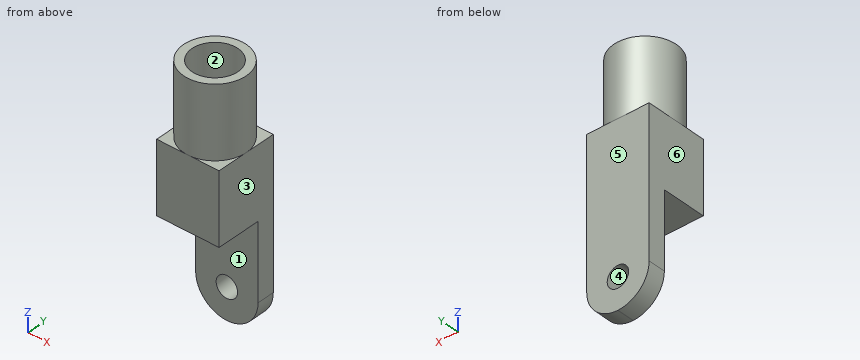
from build123d import *

# Parameters (mm, degrees)
SKETCH1_R           = 4.445
SKETCH1_R_2         = 3.275000003
BOSS_EXTRUDE1_DEPTH = 10.16
SKETCH2_W           = 8.89
SKETCH2_H           = 8.89
BOSS_EXTRUDE2_DEPTH = 25.4
CUT_EXTRUDE1_DEPTH  = 28.275449126
SKETCH4_W           = 15.24
SKETCH4_H           = 6.39064
CUT_EXTRUDE2_DEPTH  = 28.275449126


with BuildPart() as part:
    # Sketch1 → Boss-Extrude1 (new body)
    with BuildSketch(Plane.XY):
        Circle(SKETCH1_R)
        Circle(SKETCH1_R_2, mode=Mode.SUBTRACT)
    extrude(amount=BOSS_EXTRUDE1_DEPTH)

    # Sketch2 → Boss-Extrude2 (add)
    with BuildSketch(Plane(origin=(0, 0, 0), x_dir=(-1, 0, 0), z_dir=(0, 0, -1))):
        Rectangle(SKETCH2_W, SKETCH2_H)
    extrude(amount=BOSS_EXTRUDE2_DEPTH)

    # Sketch3 → Cut-Extrude1 (cut, through all)
    with BuildSketch(Plane.XZ.offset(4.445)):
        with BuildLine():
            Line((4.445, -25.4), (4.445, -20.955))
            ThreePointArc((4.445, -20.955), (3.143089642, -24.098089642), (0, -25.4))
            Line((0, -25.4), (4.445, -25.4))
        make_face()
        with BuildLine():
            ThreePointArc((0, -25.4), (-3.143089642, -24.098089642), (-4.445, -20.955))
            Line((-4.445, -20.955), (-4.445, -25.4))
            Line((-4.445, -25.4), (0, -25.4))
        make_face()
        with BuildLine():
            ThreePointArc((1.524, -20.955), (0, -19.431), (-1.524, -20.955))
            Line((-1.524, -20.955), (1.524, -20.955))
        make_face()
        with BuildLine():
            Line((1.524, -20.955), (-1.524, -20.955))
            ThreePointArc((-1.524, -20.955), (0, -22.479), (1.524, -20.955))
        make_face()
    extrude(amount=-CUT_EXTRUDE1_DEPTH, mode=Mode.SUBTRACT)

    # Sketch4 → Cut-Extrude2 (cut, through all)
    with BuildSketch(Plane.ZY.offset(4.445)):
        with Locations((-17.78, -1.24968)):
            Rectangle(SKETCH4_W, SKETCH4_H)
    extrude(amount=-CUT_EXTRUDE2_DEPTH, mode=Mode.SUBTRACT)


solid = part.part
Geometry: final body of the model. Coordinates: model frame, mm. Face numbers are marked on the shaded views. A direction names the side the tool comes from. Round coordinates to 2 decimals unless told otherwise and drop trailing zeros. Order: outer loops, then holes, each group sorted by start corner. A loop starts at its lowest first (then second) coordinate and runs counter-clockwise, first axis right, second up. Notation, with made-up numbers: (-5.75, 86.25) -> (7.25, 86.25) arc R22 cw to (7.25, 110.25) -> close; hole circle Ø5 at (29.25, -12.5). An arc over 180 degrees is marked (long way). Put each result on its own line as item: value. Start each with the question number.
Q1. Section A-A on z = 1. Return the cut outline in (x, y) (3 decimals).
Q2. Section C-C on x = 2.25. Return the cut outline in (y, z) (3 decimals), and give its area (3 significant figures).
Q3. Pull-direction query (X, two-part tool) for the marked faces 4, 5 and 6; classes: +X half, -X half, draft (parallel to the pull), parting line (faces both ways), or undercut.
Q4. Section B-B on y = 2.25. Return the cut outline in (x, z) (3 decimals).
Q5. Section D-D on y = -2. Return the cut outline in (x, z) (3 decimals).
Q6. First-contact query: pin 1 (2.5 mm diameter, centred on x = 0, z = -20.955, fed in from +Y); pin 2 (3 mm diameter, centred on x = -1.5, y = -1, fed in from -Z); pin 3 (5 mm diameter, centred on x = 3, z = -13, fed in from -Y). Flat tips, straight axial feed; report the tip coordinate or a pass-through.
Q7. Reachability of the marked faces 1, 2 and 3 from +Z, -Z, +X, -X, +Y, -Y: full face, straight path, thin tool, end or side. Return the list, or none.
Q8. Line query: probe 1 along Y at (x, z) = (0, 5.5) (3 decimals); probe 2 along Y at (x, z) = (-3, -18) (3 decimals); probe 3 along Y at (x, z) = (0.5, 7.5). Output: solid intervals per line, ascending.
Ans:
1. outline: circle Ø8.89 at (0, 0); hole circle Ø6.55 at (0, 0)
2. outline: (-4.445, -10.16) -> (1.946, -10.16) -> (1.946, -24.788) -> (4.445, -24.788) -> (4.445, 0) -> (3.833, 0) -> (3.833, 10.16) -> (2.38, 10.16) -> (2.38, 0) -> (-2.38, 0) -> (-2.38, 10.16) -> (-3.833, 10.16) -> (-3.833, 0) -> (-4.445, 0) -> close
2. area: 156 mm2
3. face 4: undercut
3. face 5: draft
3. face 6: -X half
4. outline: (-4.445, -20.955) arc R4.445 ccw to (4.445, -20.955) -> (4.445, 0) -> (3.833, 0) -> (3.833, 10.16) -> (2.38, 10.16) -> (2.38, 0) -> (-2.38, 0) -> (-2.38, 10.16) -> (-3.833, 10.16) -> (-3.833, 0) -> (-4.445, 0) -> close; hole circle Ø3.048 at (0, -20.955)
5. outline: (-4.445, -10.16) -> (4.445, -10.16) -> (4.445, 0) -> (3.97, 0) -> (3.97, 10.16) -> (2.593, 10.16) -> (2.593, 0) -> (-2.593, 0) -> (-2.593, 10.16) -> (-3.97, 10.16) -> (-3.97, 0) -> (-4.445, 0) -> close
6. pin 1: passes through
6. pin 2: stops at z = -10.16
6. pin 3: stops at y = 1.95
7. face 1: -Z, +X, -X, -Y
7. face 2: +Z
7. face 3: +Z, -Z, +X, +Y, -Y
8. probe 1: y = -4.445 to -3.275, 3.275 to 4.445
8. probe 2: y = 1.946 to 4.445
8. probe 3: y = -4.42 to -3.24, 3.24 to 4.42
